Part model, mm, in its own coordinate system. A direction names the side the tool comes from. Give positions to 0.01 mm unless a question says otherwise; leave off trailing zeros. Loops run counter-clockwise (first coordinate to the right, second up) from the corner with the lowest first, then second, coordinate; pieces in that order, holes last. Notation, with made-up numbers: M 5.25,-34 L 38.25,-34 A22 ccw 38.25,-14 Z; hole C -37,46.25 d6. An arc over 180 degrees is marked long. Answer in a Markdown table with one row per item.
from build123d import *

# Parameters (mm, degrees)
SKETCH1_R           = 0.9
SKETCH1_R_2         = 1.45
SKETCH1_R_3         = 7
SKETCH1_W           = 3.400011
SKETCH1_H           = 6.1
SKETCH1_W_2         = 3.4
BOSS_EXTRUDE2_DEPTH = 5.85


with BuildPart() as part:
    # Sketch1 → Boss-Extrude2 (new body)
    with BuildSketch(Plane.XY):
        with BuildLine():
            Line((669.21684417, 348.01545661), (648.4638119, 348.01545661))
            ThreePointArc((648.4638119, 348.01545661), (647.249496344, 347.512470637), (646.746510371, 346.298155081))
            Line((646.746510371, 346.298155081), (646.746510371, 315.232758138))
            ThreePointArc((646.746510371, 315.232758138), (647.249496344, 314.018442582), (648.4638119, 313.51545661))
            Line((648.4638119, 313.51545661), (669.21684417, 313.51545661))
            Line((669.21684417, 313.51545661), (684.726521371, 313.51545661))
            ThreePointArc((684.726521371, 313.51545661), (689.076521371, 317.86545661), (684.726521371, 322.21545661))
            Line((684.726521371, 322.21545661), (677.876521371, 322.21545661))
            ThreePointArc((677.876521371, 322.21545661), (669.326521371, 330.76545661), (677.876521371, 339.31545661))
            Line((677.876521371, 339.31545661), (684.726521371, 339.31545661))
            ThreePointArc((684.726521371, 339.31545661), (689.076521371, 343.66545661), (684.726521371, 348.01545661))
            Line((684.726521371, 348.01545661), (669.21684417, 348.01545661))
        make_face()
        with Locations((684.726521371, 343.66545661)):
            Circle(SKETCH1_R, mode=Mode.SUBTRACT)
        with Locations((684.726521371, 317.86545661)):
            Circle(SKETCH1_R, mode=Mode.SUBTRACT)
        with Locations((658.726521371, 318.56545661)):
            Circle(SKETCH1_R_2, mode=Mode.SUBTRACT)
        with Locations((658.726521371, 330.76545661)):
            Circle(SKETCH1_R_3, mode=Mode.SUBTRACT)
        with Locations((651.446515871, 342.96545661)):
            Rectangle(SKETCH1_W, SKETCH1_H, mode=Mode.SUBTRACT)
        with Locations((653.576521371, 318.56545661)):
            Rectangle(SKETCH1_W_2, SKETCH1_H, mode=Mode.SUBTRACT)
        with Locations((666.006526871, 342.96545661)):
            Rectangle(SKETCH1_W, SKETCH1_H, mode=Mode.SUBTRACT)
        with Locations((663.876521371, 318.56545661)):
            Rectangle(SKETCH1_W_2, SKETCH1_H, mode=Mode.SUBTRACT)
    extrude(amount=BOSS_EXTRUDE2_DEPTH)


solid = part.part
(1) Which spindle directions (+Z, -Z, +X, -X, +Y, -Y) get a long thin tool onto all of the face, cutting with end or side? Do faces 1 (the face through (681, 322.215, 3)), 2 (the face through (651, 339.915, 3)). Say none if no direction does.
Recorded:
| item | result |
|---|---|
| face 1 | +Z, -Z, +X |
| face 2 | +Z, -Z |
(2) Pin check, flat tips, straight feed: pin 1 Ø1.4 at (x, y) = (684.73, 317.87) entering from -Z; pin 2 Ø2 at (y, z) = (336, 2.5) entering from +X. Stop position of each tip, or through.
Recorded:
| item | result |
|---|---|
| pin 1 | passes through |
| pin 2 | stops at x = 672.03 |
(3) Saw through at A-A (y = 341). Write the cut outline in (x, z), plus the area to 3 significant figures.
Recorded:
| item | result |
|---|---|
| outline | M 646.75,0 L 649.75,0 L 649.75,5.85 L 646.75,5.85 Z; M 653.15,0 L 664.31,0 L 664.31,5.85 L 653.15,5.85 Z; M 667.71,0 L 688.16,0 L 688.16,5.85 L 667.71,5.85 Z |
| area | 203 mm^2 |
(4) Saw through at D-D (x = 683). Write the cut outline in (y, z), plus the area to 3 significant figures.
Recorded:
| item | result |
|---|---|
| outline | M 313.52,0 L 322.22,0 L 322.22,5.85 L 313.52,5.85 Z; M 339.32,0 L 348.02,0 L 348.02,5.85 L 339.32,5.85 Z |
| area | 102 mm^2 |
(5) Drill centre lines: line 1 along Y through (x, z) = (682.5, 5.4); line 2 along X through (y, z) = (341.5, 4.2); line 3 along Y through (x, z) = (685, 4.1). Where is each one in solid material? Low to high.
Recorded:
| item | result |
|---|---|
| line 1 | y = 313.52 to 322.22, 339.32 to 348.02 |
| line 2 | x = 646.75 to 649.75, 653.15 to 664.31, 667.71 to 688.5 |
| line 3 | y = 313.52 to 317.01, 318.72 to 322.21, 339.32 to 342.81, 344.52 to 348.01 |
(6) Saw through at C-C (y = 333). Write the cut outline in (x, z).
Recorded:
| item | result |
|---|---|
| outline | M 646.75,0 L 652.09,0 L 652.09,5.85 L 646.75,5.85 Z; M 665.36,0 L 669.62,0 L 669.62,5.85 L 665.36,5.85 Z |
(7) Saw through at B-B (x = 658). Write the cut outline in (y, z), plus the area to 3 significant figures.
Recorded:
| item | result |
|---|---|
| outline | M 313.52,0 L 317.31,0 L 317.31,5.85 L 313.52,5.85 Z; M 319.82,0 L 323.8,0 L 323.8,5.85 L 319.82,5.85 Z; M 337.73,0 L 348.02,0 L 348.02,5.85 L 337.73,5.85 Z |
| area | 106 mm^2 |
(8) Pull direction Y, two halves, no side cores. Call faces 3 (the face through (683.827, 317.905, 2.884)), 4 (the face through (668, 331, 5.85)), 5 (the face through (647.263, 347.526, 2.884)): +Y half, -Y half, draft (parallel to the pull), parting line (faces both ways), or undercut.
Recorded:
| item | result |
|---|---|
| face 3 | undercut |
| face 4 | draft |
| face 5 | +Y half |
